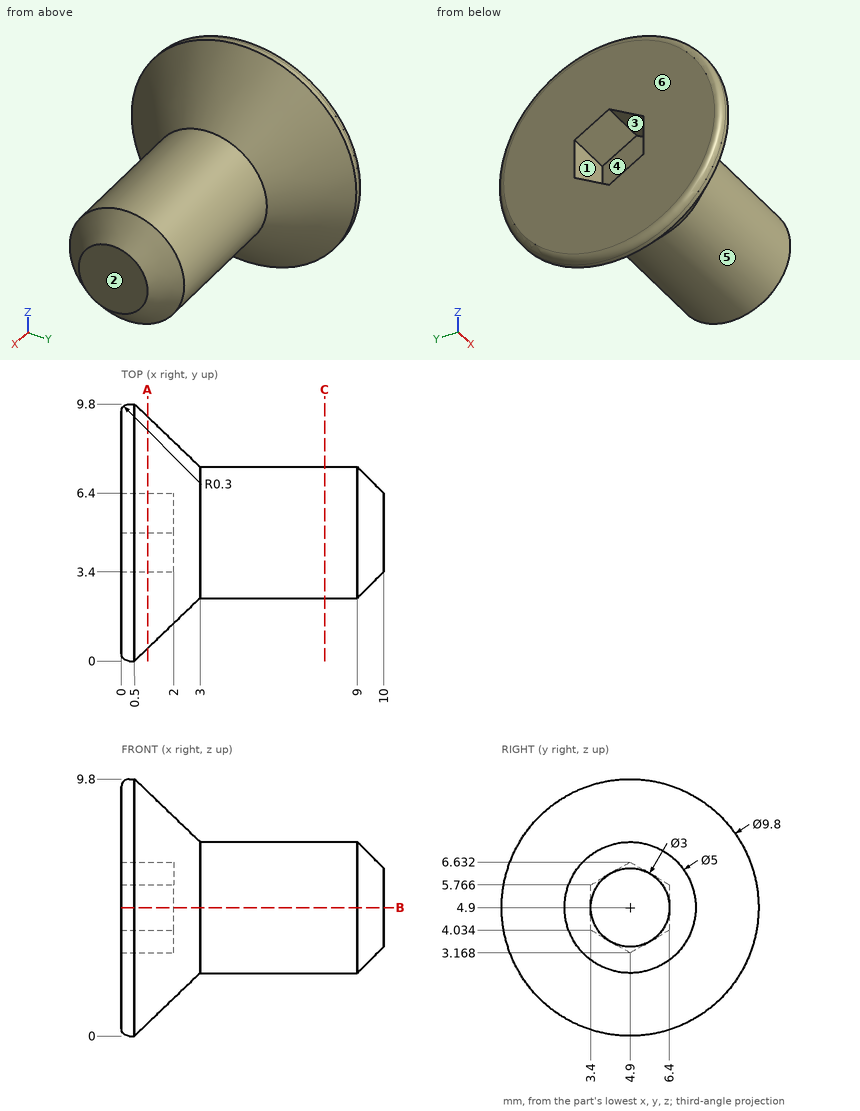
The figure shows three views and two pictorial views of one solid part (mm, origin at its lowest corner). Answer the questions. A direction names the side the tool comes from. Coordinates: 2 decimals unless noted, no trailing zeros. Order: outer loops, then holes, each group sorted by start corner. A loop starts at its lowest first (then second) coordinate and runs counter-clockwise, first axis right, second up.
Q1. A cutting plane is placed at B-B, the plane z = 4.9. Write down the section's boundary in (x, y), and give its area (3 significant figures).
Q2. For a pull along Y with two mould halves and no side action, classify the marked faces 3, 4, 5 and 6 as pulls with the +Y half, pulls with the -Y half, needs draft (parallel to the pull), parting line crosses it, or undercut.
Q3. A cutting plane is placed at A-A, the plane x = 1. Write down the section's boundary in (y, z).
Q4. Which of the six approach directions +Z, -Z, +X, -X, +Y, -Y give full straight-line access (tool end or side, diameter ignored) to the marked faces 1 and 2?
Q5. A cutting plane is placed at C-C, the plane x = 7.75. Write down the section's boundary in (y, z), and give its area (3 significant figures).
Q6. Given P1, Ø1, axis at y = 8, z = 4.5, coming from the +X side; P2, Ø1.5, axis at y = 1, z = 5.5, coming from the +X side (3 decimals), each flat-ended and moving along its own axis, determine where each tip first touches the part or whether it passes through.
Q7. Consider line 1 (X direction, y = 5, z = 5.5); line 2 (X direction, y = 6, z = 8); line 3 (Z direction, x = 6.75, y = 4.75). Determine where each line is inside the solid, lowest interval first.
Answers follow:
1. outline: (0, 0.3) arc R0.3 ccw to (0.3, 0) - (0.5, 0) - (3, 2.4) - (9, 2.4) - (10, 3.4) - (10, 6.4) - (9, 7.4) - (3, 7.4) - (0.5, 9.8) - (0.3, 9.8) arc R0.3 ccw to (0, 9.5) - (0, 6.4) - (2, 6.4) - (2, 3.4) - (0, 3.4) - close
1. area: 51.4 mm2
2. face 3: undercut
2. face 4: undercut
2. face 5: parting line crosses it
2. face 6: needs draft
3. outline: circle Ø8.84 at (4.9, 4.9); hole (3.4, 4.03) - (4.9, 3.17) - (6.4, 4.03) - (6.4, 5.77) - (4.9, 6.63) - (3.4, 5.77) - close
4. face 1: -X
4. face 2: +Z, -Z, +X, +Y, -Y
5. outline: circle Ø5 at (4.9, 4.9)
5. area: 19.6 mm2
6. P1: stops at x = 2.87
6. P2: stops at x = 2.275
7. line 1: x = 2 to 10
7. line 2: x = 0 to 2.18
7. line 3: z = 2.4 to 7.4
